Geometry check sheet. Reference: drawing and pictorial views, mm from the part's lowest x, y, z. A direction names the side the tool comes from. Coordinates: 2 decimals unless noted, no trailing zeros. Write each loop counter-clockwise with the first axis right and the second up, starting at its lowest first coordinate (ties: lowest second). Pieces come first, ordered by that corner, then holes. Notation, with made-up numbers: M 12,-37.5 L 59,-37.5 A21 ccw 59,-4.5 Z; hole C 6,-7 d8. An arc over 180 degrees is marked long. One line per item, written item: value.
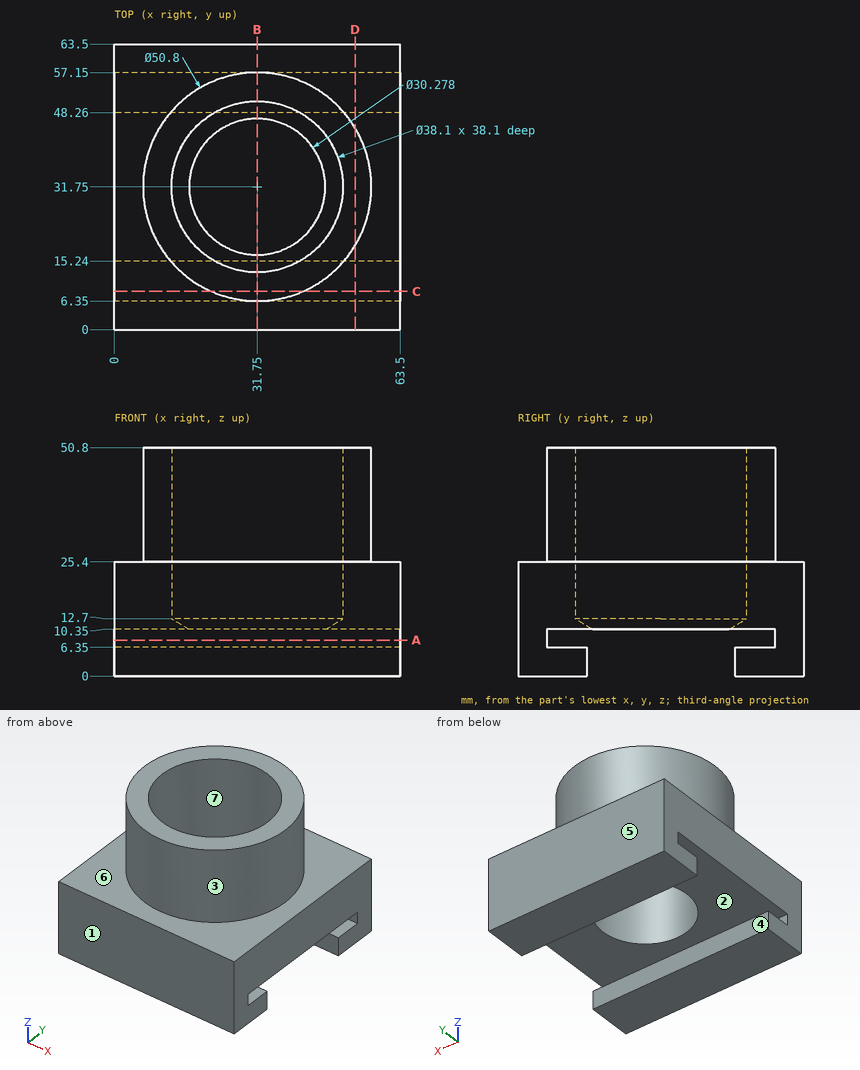
Item 1: Scan lines: line 1 (Z direction, x = 22, y = 9); line 2 (Y direction, x = 31.75, z = 30); line 3 (Y direction, x = 31.75, z = 24). Record each from-to range of solid material in increasing order.
The answers:
line 1: z = 0 to 6.35, 10.35 to 50.8
line 2: y = 6.35 to 12.7, 50.8 to 57.15
line 3: y = 0 to 12.7, 50.8 to 63.5
Item 2: Cross-section at A-A, the plane z = 8. Enter the section's corners in (x, y).
The answers:
outline: M 0,0 L 63.5,0 L 63.5,6.35 L 0,6.35 Z; M 0,57.15 L 63.5,57.15 L 63.5,63.5 L 0,63.5 Z
Item 3: Go/stop test with flat-tipped pins: P1, Ø1, axis at y = 53.5, z = 6.5, coming from the +X side; P2, Ø12, axis at x = 51, z = 40.5, coming from the +Y side; P3, Ø10, axis at y = 25.5, z = 37, coming from the +X side; P4, Ø10, axis at x = 16.5, z = 38, coming from the -Y side. Record where each tip stops, or that it passes through.
The answers:
P1: stops at x = 63.5
P2: stops at y = 53.42
P3: stops at x = 57.12
P4: stops at y = 8.51
Item 4: Cross-section at C-C, the plane y = 8.5. Enter the section's corners in (x, z), and give its area (3 significant figures).
The answers:
outline: M 0,0 L 63.5,0 L 63.5,6.35 L 0,6.35 Z; M 0,10.35 L 63.5,10.35 L 63.5,25.4 L 41.98,25.4 L 41.98,50.8 L 21.52,50.8 L 21.52,25.4 L 0,25.4 Z
area: 1,880 mm²
Item 5: Access from +Z, -Z, +X, -X, +Y, -Y to the whole of each face (thin tool, end or side, straight path). Record for the marked faces 1, 2, 3 and 4.
The answers:
face 1: +Z, -Z, +X, -X, -Y
face 2: +X, -X
face 3: +Z
face 4: -Z, +X, -X
Item 6: Cross-section at B-B, the plane x = 31.75. Enter the section's corners in (y, z).
The answers:
outline: M 0,0 L 15.24,0 L 15.24,6.35 L 6.35,6.35 L 6.35,10.35 L 16.61,10.35 L 12.7,12.7 L 12.7,50.8 L 6.35,50.8 L 6.35,25.4 L 0,25.4 Z; M 46.89,10.35 L 57.15,10.35 L 57.15,6.35 L 48.26,6.35 L 48.26,0 L 63.5,0 L 63.5,25.4 L 57.15,25.4 L 57.15,50.8 L 50.8,50.8 L 50.8,12.7 Z
Item 7: Cross-section at D-D, the plane x = 53.5. Enter the section's corners in (y, z).
The answers:
outline: M 0,0 L 15.24,0 L 15.24,6.35 L 6.35,6.35 L 6.35,10.35 L 57.15,10.35 L 57.15,6.35 L 48.26,6.35 L 48.26,0 L 63.5,0 L 63.5,25.4 L 44.87,25.4 L 44.87,50.8 L 18.63,50.8 L 18.63,25.4 L 0,25.4 Z
Item 8: Draft check along Y on the marked faces 5, 6 and 7. Enter one of: released by +Y, released by -Y, zero draft, split by the parting line, or undercut.
The answers:
face 5: released by +Y
face 6: zero draft
face 7: undercut
